```python
from build123d import *

# Parameters (mm, degrees)
SKETCH1_W           = 145
SKETCH1_H           = 35
SKETCH1_W_2         = 1
SKETCH1_H_2         = 3.6
BOSS_EXTRUDE1_DEPTH = 5
CUT_EXTRUDE1_REACH  = 76.75
SKETCH2_W           = 145
SKETCH2_H           = 13.752262189
SKETCH2_W_2         = 62.00633413
SKETCH2_H_2         = 13.452443164
SKETCH4_R           = 1.9
CUT_EXTRUDE2_DEPTH  = 3


with BuildPart() as part:
    # Sketch1 → Boss-Extrude1 (new body)
    with BuildSketch(Plane(origin=(0, 0, 0), x_dir=(1, 0, 0), z_dir=(0, 1, 0))):
        Rectangle(SKETCH1_W, SKETCH1_H)
        Rectangle(SKETCH1_W_2, SKETCH1_H_2, mode=Mode.SUBTRACT)
        with Locations((-22.72, 0)):
            Rectangle(SKETCH1_W_2, SKETCH1_H_2, mode=Mode.SUBTRACT)
        with Locations((-33.595, 0)):
            Rectangle(SKETCH1_W_2, SKETCH1_H_2, mode=Mode.SUBTRACT)
        with Locations((-44.47, 0)):
            Rectangle(SKETCH1_W_2, SKETCH1_H_2, mode=Mode.SUBTRACT)
        with Locations((-55.345, 0)):
            Rectangle(SKETCH1_W_2, SKETCH1_H_2, mode=Mode.SUBTRACT)
        with Locations((-66.22, 0)):
            Rectangle(SKETCH1_W_2, SKETCH1_H_2, mode=Mode.SUBTRACT)
        with Locations((22.7, 0)):
            Rectangle(SKETCH1_W_2, SKETCH1_H_2, mode=Mode.SUBTRACT)
        with Locations((33.337, 0)):
            Rectangle(SKETCH1_W_2, SKETCH1_H_2, mode=Mode.SUBTRACT)
        with Locations((44.499, 0)):
            Rectangle(SKETCH1_W_2, SKETCH1_H_2, mode=Mode.SUBTRACT)
        with Locations((55.661, 0)):
            Rectangle(SKETCH1_W_2, SKETCH1_H_2, mode=Mode.SUBTRACT)
        with Locations((66.298, 0)):
            Rectangle(SKETCH1_W_2, SKETCH1_H_2, mode=Mode.SUBTRACT)
        with Locations((-5.4, 12.38)):
            Rectangle(SKETCH1_W_2, SKETCH1_H_2, mode=Mode.SUBTRACT)
        with Locations((5.4, 12.38)):
            Rectangle(SKETCH1_W_2, SKETCH1_H_2, mode=Mode.SUBTRACT)
        with Locations((28.019, 12.38)):
            Rectangle(SKETCH1_W_2, SKETCH1_H_2, mode=Mode.SUBTRACT)
        with Locations((38.918, 12.38)):
            Rectangle(SKETCH1_W_2, SKETCH1_H_2, mode=Mode.SUBTRACT)
        with Locations((60.717, 12.38)):
            Rectangle(SKETCH1_W_2, SKETCH1_H_2, mode=Mode.SUBTRACT)
    extrude(amount=BOSS_EXTRUDE1_DEPTH)

    # Sketch2 → Cut-Extrude1 (cut, up to next)
    with BuildSketch(Plane(origin=(0, 5, 0), x_dir=(1, 0, 0), z_dir=(0, 1, 0)), mode=Mode.PRIVATE) as cut_extrude1_sk1:
        with Locations((0, -10.623868906)):
            Rectangle(SKETCH2_W, SKETCH2_H)
    cut_extrude1_tool1 = extrude(cut_extrude1_sk1.sketch, amount=-CUT_EXTRUDE1_REACH, mode=Mode.PRIVATE) & part.part
    # Sketch2 → Cut-Extrude1 (cut, up to next)
    with BuildSketch(Plane(origin=(0, 5, 0), x_dir=(1, 0, 0), z_dir=(0, 1, 0)), mode=Mode.PRIVATE) as cut_extrude1_sk2:
        with Locations((-41.496832935, 10.773778418)):
            Rectangle(SKETCH2_W_2, SKETCH2_H_2)
    cut_extrude1_tool2 = extrude(cut_extrude1_sk2.sketch, amount=-CUT_EXTRUDE1_REACH, mode=Mode.PRIVATE) & part.part
    add(cut_extrude1_tool1.solids().sort_by_distance((0, 5, 10.623869))[0], mode=Mode.SUBTRACT)
    add(cut_extrude1_tool2.solids().sort_by_distance((-41.496833, 5, -10.773778))[0], mode=Mode.SUBTRACT)

    # Sketch4 → Cut-Extrude2 (cut)
    with BuildSketch(Plane.XZ):
        with Locations(Location((0, 0, 0), (0, 0, 270))):
            Circle(SKETCH4_R)
        with Locations(Location((-5.4, -12.38, 0), (0, 0, 270))):
            Circle(SKETCH4_R)
        with Locations(Location((-22.72, 0, 0), (0, 0, 270))):
            Circle(SKETCH4_R)
        with Locations(Location((-33.595, 0, 0), (0, 0, 270))):
            Circle(SKETCH4_R)
        with Locations(Location((-44.47, 0, 0), (0, 0, 270))):
            Circle(SKETCH4_R)
        with Locations(Location((-55.345, 0, 0), (0, 0, 270))):
            Circle(SKETCH4_R)
        with Locations(Location((-66.22, 0, 0), (0, 0, 270))):
            Circle(SKETCH4_R)
        with Locations(Location((5.4, -12.38, 0), (0, 0, 270))):
            Circle(SKETCH4_R)
        with Locations(Location((22.7, 0, 0), (0, 0, 270))):
            Circle(SKETCH4_R)
        with Locations(Location((33.337, 0, 0), (0, 0, 270))):
            Circle(SKETCH4_R)
        with Locations(Location((44.499, 0, 0), (0, 0, 270))):
            Circle(SKETCH4_R)
        with Locations(Location((55.661, 0, 0), (0, 0, 270))):
            Circle(SKETCH4_R)
        with Locations(Location((66.298, 0, 0), (0, 0, 270))):
            Circle(SKETCH4_R)
        with Locations(Location((28.019, -12.38, 0), (0, 0, 270))):
            Circle(SKETCH4_R)
        with Locations(Location((38.918, -12.38, 0), (0, 0, 270))):
            Circle(SKETCH4_R)
        with Locations(Location((60.717, -12.38, 0), (0, 0, 270))):
            Circle(SKETCH4_R)
    extrude(amount=-CUT_EXTRUDE2_DEPTH, mode=Mode.SUBTRACT)


solid = part.part
```
The listing builds one solid part. Answer for the finished solid, in the listing's coordinates (mm). A direction names the side the tool comes from. Coordinates: 2 decimals unless noted, no trailing zeros. Loops run counter-clockwise (first coordinate to the right, second up) from the corner with the lowest first, then second, coordinate; pieces in that order, holes last. Notation, with made-up numbers: (88.5, 74) - (108.5, 74) arc R14 ccw to (108.5, 101) - close; hole circle Ø6 at (15, 87.25). An arc over 180 degrees is marked (long way). Use a Markdown table: item, result. Add a question column.
1) Find the intervals of material crossed by line 1 (X direction, y = 2.35, z = -12.38); line 2 (X direction, y = 0.55, z = -13) (3 decimals); line 3 (Z direction, x = 6, y = 0.75), in increasing order.
2) The mould has two halves that part along Z. Classify faces 1 (the flat face through (-42, 3, -4.048)), 2 (the cylindrical face through (53.806, 1.479, 0.412)), 3 (the flat face through (-10.494, 3, -11)): released by +Z, released by -Z, zero draft, split by the parting line, or undercut.
3) Given pin 1 (3.5 mm diameter, centred on x = 28.019, z = -12.38, fed in from -Y); pin 2 (1.5 mm diameter, centred on y = 4, z = -5.5, fed in from -X), each flat-ended and moving along its own axis, determine where each tip first touches the part or whether it passes through.
4) The part is cut by section A-A, the plane z = 0. State how many separate pieces and enclosed holes the cut face has, and give its area (3 significant figures).
5) For faces 4 (the flat face through (15, 0, -7)), 5 (the flat face through (4.6, 3, -12.4)), determine the directions among +Z, -Z, +X, -X, +Y, -Y from which every point of the face is accessible in a straight line to the end or side of a thin tool.
6) The part is cut by section D-D, the plane x = -16.5. Give the vertices of the cut face in (y, z).
Here are the results:
| question | item | result |
|---|---|---|
| 1 | line 1 | x = -10.49 to -7.3, -3.5 to 3.5, 7.3 to 26.12, 29.92 to 37.02, 40.82 to 58.82, 62.62 to 72.5 |
| 1 | line 2 | x = -10.494 to -7.196, -3.604 to 3.604, 7.196 to 26.223, 29.815 to 37.122, 40.714 to 58.921, 62.513 to 72.5 |
| 1 | line 3 | z = -17.5 to -14.18, -10.58 to 3.75 |
| 2 | face 1 | released by -Z |
| 2 | face 2 | undercut |
| 2 | face 3 | zero draft |
| 3 | pin 1 | stops at y = 3 |
| 3 | pin 2 | stops at x = -10.49 |
| 4 | separate pieces | 12 |
| 4 | enclosed holes | 0 |
| 4 | area | 578 mm^2 |
| 5 | face 4 | +Z, -Z, +X, -X, -Y |
| 5 | face 5 | -Y |
| 6 | outline | (0, -4.05) - (5, -4.05) - (5, 3.75) - (0, 3.75) - close |
